Here's the drawing with two shaded views (mm, measured from the low corner). I have some questions. A direction names the side the tool comes from. Coordinates: 2 decimals unless noted, no trailing zeros. Write each loop counter-clockwise with the first axis right and the second up, starting at its lowest first coordinate (ties: lowest second). Pieces come first, ordered by that corner, then holes. Notation, with made-up numbers: (-38, 52.5) -> (19, 52.5) arc R17 ccw to (19, 61.5) -> close; hole circle Ø8 at (70.5, 59). An arc over 180 degrees is marked (long way). Put each result on its own line as item: value. Start each with the question number.
Item 1: I want a section at A-A, the plane x = 10. List the corners of the cut face in (y, z) for me (1 decimal).
Item 2: If we mould it in two halves opening along Y, with no side actions, what happens to the marked faces 1, 2, 3 and 4? For each: released by +Y, released by -Y, zero draft, split by the parting line, or undercut.
Item 3: I want a section at D-D, the plane y = 11. List the corners of the cut face in (x, z) for me.
Item 4: For pin 1 (6 mm diameter, centred on x = 13, y = 31.5, fed in from +Z), with a flat end and sliding along its axis, tell me the tip position at first contact or that it passes through.
Item 5: On a 3-axis mill with a long thin cutter (end or side, diameter ignored), from which of +Z, -Z, +X, -X, +Y, -Y can I reach the whole of each face in a straight line? I mean the marked faces 5 and 6. Say none if no direction works.
Item 6: I want a section at C-C, the plane x = 14.5. List the corners of the cut face in (y, z) for me.
Item 7: I need wall thicknesses on line 1 (Y direction, x = 11.5, z = 18); line 2 (Z direction, x = 18.5, y = 9); line 3 (Z direction, x = 9.75, y = 4). Which ranges of each line are inside material? Lowest first, please. Write a range as [from, to].
Item 8: I want a section at B-B, the plane z = 27. List the corners of the cut face in (x, y) for me.
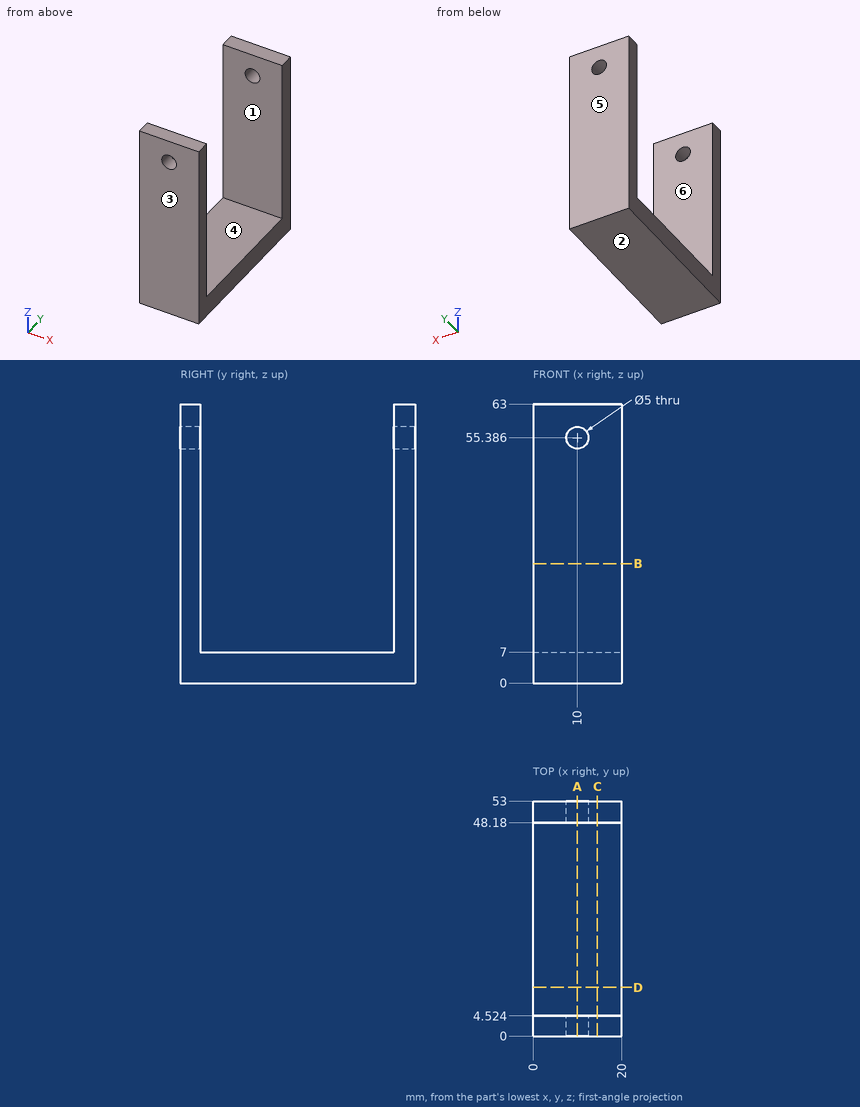
Calculated:
1. outline: (0, 0) -> (53, 0) -> (53, 52.9) -> (48.2, 52.9) -> (48.2, 7) -> (4.5, 7) -> (4.5, 52.9) -> (0, 52.9) -> close; (0, 57.9) -> (4.5, 57.9) -> (4.5, 63) -> (0, 63) -> close; (48.2, 57.9) -> (53, 57.9) -> (53, 63) -> (48.2, 63) -> close
2. face 1: undercut
2. face 2: zero draft
2. face 3: released by -Y
2. face 4: undercut
3. outline: (0, 0) -> (20, 0) -> (20, 7) -> (0, 7) -> close
4. pin 1: stops at z = 7
5. face 5: +Z, -Z, +X, -X, +Y
5. face 6: +Z, +X, -X
6. outline: (0, 0) -> (53, 0) -> (53, 63) -> (48.18, 63) -> (48.18, 7) -> (4.52, 7) -> (4.52, 63) -> (0, 63) -> close
7. line 1: y = [0, 4.52], [48.18, 53]
7. line 2: z = [0, 7]
7. line 3: z = [0, 52.9], [57.87, 63]
8. outline: (0, 0) -> (20, 0) -> (20, 4.52) -> (0, 4.52) -> close; (0, 48.18) -> (20, 48.18) -> (20, 53) -> (0, 53) -> close
